from build123d import *

# Parameters (mm, degrees)
BOSS_EXTRUDE1_DEPTH = 355.6
SKETCH2_R           = 3.429
SKETCH2_R_2         = 14.2875
CUT_EXTRUDE1_DEPTH  = 26.4
SKETCH3_R           = 3.429
CUT_EXTRUDE2_DEPTH  = 26.4


with BuildPart() as part:
    # Sketch1 → Boss-Extrude1 (new body)
    with BuildSketch(Plane(origin=(0, 0, 0), x_dir=(1, 0, 0), z_dir=(0, 1, 0))):
        with BuildLine():
            Line((-12.446, -25.4), (12.446, -25.4))
            ThreePointArc((12.446, -25.4), (12.625605122, -25.325605122), (12.7, -25.146))
            Line((12.7, -25.146), (12.7, 25.146))
            ThreePointArc((12.7, 25.146), (12.625605122, 25.325605122), (12.446, 25.4))
            Line((12.446, 25.4), (-12.446, 25.4))
            ThreePointArc((-12.446, 25.4), (-12.625605122, 25.325605122), (-12.7, 25.146))
            Line((-12.7, 25.146), (-12.7, -25.146))
            ThreePointArc((-12.7, -25.146), (-12.625605122, -25.325605122), (-12.446, -25.4))
        make_face()
        with BuildLine():
            Line((-9.5885, 23.8125), (9.5885, 23.8125))
            ThreePointArc((9.5885, 23.8125), (10.666130735, 23.366130735), (11.1125, 22.2885))
            Line((11.1125, 22.2885), (11.1125, -22.2885))
            ThreePointArc((11.1125, -22.2885), (10.666130735, -23.366130735), (9.5885, -23.8125))
            Line((9.5885, -23.8125), (-9.5885, -23.8125))
            ThreePointArc((-9.5885, -23.8125), (-10.666130735, -23.366130735), (-11.1125, -22.2885))
            Line((-11.1125, -22.2885), (-11.1125, 22.2885))
            ThreePointArc((-11.1125, 22.2885), (-10.666130735, 23.366130735), (-9.5885, 23.8125))
        make_face(mode=Mode.SUBTRACT)
    extrude(amount=BOSS_EXTRUDE1_DEPTH)

    # Sketch2 → Cut-Extrude1 (cut, through all)
    with BuildSketch(Plane.ZY.offset(12.7)):
        with Locations((-8.632581672, 35.844574716)):
            Circle(SKETCH2_R)
        with Locations((0, 330.2)):
            Circle(SKETCH2_R_2)
        with Locations((0, 292.1)):
            Circle(SKETCH2_R)
        with Locations((12.7, 292.1)):
            Circle(SKETCH2_R)
        with Locations((-12.7, 292.1)):
            Circle(SKETCH2_R)
        with Locations((2.877527224, 41.21182664)):
            Circle(SKETCH2_R)
        with Locations((14.387636119, 46.579078564)):
            Circle(SKETCH2_R)
        with Locations((-2.4897247, 52.721935535)):
            Circle(SKETCH2_R)
        with Locations((9.020384195, 58.089187459)):
            Circle(SKETCH2_R)
        with Locations((-13.999833596, 47.354683611)):
            Circle(SKETCH2_R)
        with Locations((12.7, 190.5)):
            Circle(SKETCH2_R)
        with Locations((12.7, 88.9)):
            Circle(SKETCH2_R)
        Polygon((-25.4, 0), (25.4, 23.688429034), (25.4, 0), align=None)
    extrude(amount=-CUT_EXTRUDE1_DEPTH, mode=Mode.SUBTRACT)

    # Sketch3 → Cut-Extrude2 (cut, through all)
    with BuildSketch(Plane.XY):
        with Locations((0, 177.8)):
            Circle(SKETCH3_R)
        with Locations((0, 120.65)):
            Circle(SKETCH3_R)
    extrude(amount=CUT_EXTRUDE2_DEPTH, mode=Mode.SUBTRACT)


solid = part.part
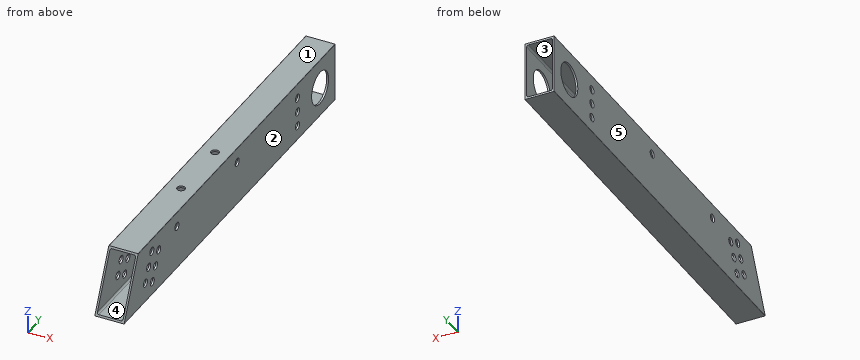
For this review, take the finished solid that the model builds, in its own axes (mm). Face numbers are marked on the shaded views. A direction names the side the tool comes from. Coordinates: 2 decimals unless noted, no trailing zeros. Loops run counter-clockwise (first coordinate to the right, second up) from the corner with the lowest first, then second, coordinate; pieces in that order, holes last. Notation, with made-up numbers: (86.5, 17.25) -> (92.5, 17.25) arc R31 ccw to (92.5, 46.25) -> close; hole circle Ø4 at (61.5, 36.25). An arc over 180 degrees is marked (long way). Write each question's results on one line, items separated by ' | '.
Q1. Machinability: for the marked faces 4 and 5, which of the approach directions +Z, -Z, +X, -X, +Y, -Y give a long, thin tool a straight path to every point of the face, cutting with its end or side? Answer none if there is none.
Taken from the geometry:
face 4: +Y, -Y | face 5: +Z, -Z, -X, +Y, -Y
Q2. Add section B-B, the plane x = 0. State the section outline as (y, z) points, then the cut area to 3 significant figures.
Taken from the geometry:
outline: (0, -25.4) -> (355.6, -25.4) -> (355.6, -23.81) -> (0.74, -23.81) -> close; (22.95, 23.81) -> (117.22, 23.81) -> (117.22, 25.4) -> (23.69, 25.4) -> close; (124.08, 23.81) -> (174.37, 23.81) -> (174.37, 25.4) -> (124.08, 25.4) -> close; (181.23, 23.81) -> (355.6, 23.81) -> (355.6, 25.4) -> (181.23, 25.4) -> close | area: 1,070 mm²
Q3. Add section A-A, the plane y = 190.5. State the section outline as (x, z) points, then the cut area to 3 significant figures.
Taken from the geometry:
outline: (-12.7, -25.15) arc R0.25 ccw to (-12.45, -25.4) -> (12.45, -25.4) arc R0.25 ccw to (12.7, -25.15) -> (12.7, 9.27) -> (11.11, 9.27) -> (11.11, -22.29) arc R1.52 cw to (9.59, -23.81) -> (-9.59, -23.81) arc R1.52 cw to (-11.11, -22.29) -> (-11.11, 9.27) -> (-12.7, 9.27) -> close; (-12.7, 16.13) -> (-11.11, 16.13) -> (-11.11, 22.29) arc R1.52 cw to (-9.59, 23.81) -> (9.59, 23.81) arc R1.52 cw to (11.11, 22.29) -> (11.11, 16.13) -> (12.7, 16.13) -> (12.7, 25.15) arc R0.25 ccw to (12.45, 25.4) -> (-12.45, 25.4) arc R0.25 ccw to (-12.7, 25.15) -> close | area: 212 mm²
Q4. To check wall thickness, follow line 1 along X through (y, z) = (251.5, 7.5); line 2 along Z through (x, y) = (1.5, 26); line 3 along Y through (x, z) = (-12.2, -12.7). State the ranges of each line that lie inside material, in increasing order. Write a range as [from, to].
Taken from the geometry:
line 1: [-12.7, -11.11], [11.11, 12.7] | line 2: [-25.4, -23.81], [23.81, 25.4] | line 3: [5.92, 44.18], [50.53, 288.67], [295.53, 323.65], [336.75, 355.6]
Q5. Mouldability with a two-part tool opening along Z and no side actions: class the marked faces 1, 2 and 3 as +Z half, -Z half, draft (parallel to the pull), parting line (faces both ways), or undercut.
Taken from the geometry:
face 1: +Z half | face 2: draft | face 3: undercut
Q6. For pin 1 Ø10 at (x, z) = (8, 6.5) entering from -Y, flat-tipped, find the tip position at first contact; note if it passes through.
Taken from the geometry:
pin 1: y = 13.05
Q7. Add section C-C, the plane y = 120.65. State the section outline as (x, z) points.
Taken from the geometry:
outline: (-12.7, -25.15) arc R0.25 ccw to (-12.45, -25.4) -> (12.45, -25.4) arc R0.25 ccw to (12.7, -25.15) -> (12.7, 25.15) arc R0.25 ccw to (12.45, 25.4) -> (3.43, 25.4) -> (3.43, 23.81) -> (9.59, 23.81) arc R1.52 cw to (11.11, 22.29) -> (11.11, -22.29) arc R1.52 cw to (9.59, -23.81) -> (-9.59, -23.81) arc R1.52 cw to (-11.11, -22.29) -> (-11.11, 22.29) arc R1.52 cw to (-9.59, 23.81) -> (-3.43, 23.81) -> (-3.43, 25.4) -> (-12.45, 25.4) arc R0.25 ccw to (-12.7, 25.15) -> close
